Here's how the part is built. I have some questions about the finished solid (model axes, mm). Face numbers are marked on the shaded views. A direction names the side the tool comes from. Round coordinates to 2 decimals unless told otherwise and drop trailing zeros. Order: outer loops, then holes, each group sorted by start corner. A loop starts at its lowest first (then second) coordinate and runs counter-clockwise, first axis right, second up.
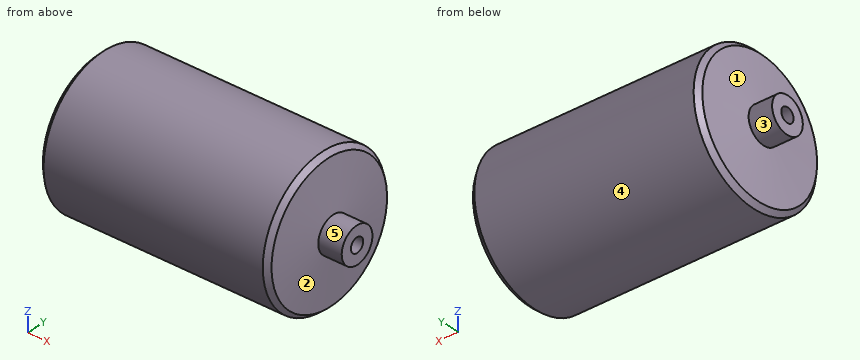
```python
from build123d import *
from OCP.BRepFilletAPI import BRepFilletAPI_MakeChamfer

# Parameters (mm, degrees)
CHAMFER1_SIZE              = 3
CHAMFER1_SIZE2             = 3.300188603
F_10_0MM_DOWEL_HOLE1_D     = 10
F_10_0MM_DOWEL_HOLE1_DEPTH = 59
F_10_0MM_DOWEL_HOLE1_TIP   = 3.004303095
F_10_0MM_DOWEL_HOLE2_D     = 10
F_10_0MM_DOWEL_HOLE2_DEPTH = 59
F_10_0MM_DOWEL_HOLE2_TIP   = 3.004303095


with BuildPart() as part:
    # Sketch1 → Revolve1 (revolve)
    with BuildSketch(Plane.XY, mode=Mode.PRIVATE) as revolve1_sk:
        Polygon((-96.096096096, 28.340840841), (103.903903904, 28.340840841), (103.903903904, 40.840840841), (87.403903904, 40.840840841), (84.123079022, 78.340840841), (-76.315271214, 78.340840841), (-79.596096096, 40.840840841), (-96.096096096, 40.840840841), align=None)
    revolve(revolve1_sk.sketch.rotate(Axis((-96.096096096, 28.340840841, 0), (1, 0, 0)), 90), axis=Axis((-96.096096096, 28.340840841, 0), (1, 0, 0)))

    # Chamfer1: one chamfer whose edges measure the first distance from different faces: ONE call of the kernel's chamfer builder (chamfer() names one face for all edges)
    chamfer1_edges_1 = [part.edges().sort_by_distance(p)[0] for p in [
        (-76.315271214, 28.340840841, -50),
    ]]
    chamfer1_side_1 = [part.faces().sort_by_distance(p)[0] for p in [
        (3.903903904, 28.340840841, -50),
    ]]
    chamfer1_edges_2 = [part.edges().sort_by_distance(p)[0] for p in [
        (84.123079022, 28.340840841, -50),
    ]]
    chamfer1_side_2 = [part.faces().sort_by_distance(p)[0] for p in [
        (85.763491463, 28.340840841, -31.25),
    ]]
    chamfer1 = BRepFilletAPI_MakeChamfer(part.part.solid().wrapped)
    for e in chamfer1_edges_1:
        chamfer1.Add(CHAMFER1_SIZE, CHAMFER1_SIZE2, e.wrapped, chamfer1_side_1[0].wrapped)  # the first distance lies on this face
    for e in chamfer1_edges_2:
        chamfer1.Add(CHAMFER1_SIZE, CHAMFER1_SIZE2, e.wrapped, chamfer1_side_2[0].wrapped)  # the first distance lies on this face
    add(Compound.cast(chamfer1.Shape()), mode=Mode.REPLACE)

    # 10.0mm Dowel Hole1
    with Locations(Plane(origin=(103.903903904, 0, 0), x_dir=(0, 0, -1), z_dir=(1, 0, 0))):
        with Locations((0, 28.340840841)):
            Hole(F_10_0MM_DOWEL_HOLE1_D / 2, depth=F_10_0MM_DOWEL_HOLE1_DEPTH)
            with Locations((0, 0, -(F_10_0MM_DOWEL_HOLE1_DEPTH + F_10_0MM_DOWEL_HOLE1_TIP / 2))):  # 118° drill point
                Cone(0, F_10_0MM_DOWEL_HOLE1_D / 2, F_10_0MM_DOWEL_HOLE1_TIP, mode=Mode.SUBTRACT)

    # 10.0mm Dowel Hole2
    with Locations(Plane.ZY.offset(96.096096096)):
        with Locations((0, 28.340840841)):
            Hole(F_10_0MM_DOWEL_HOLE2_D / 2, depth=F_10_0MM_DOWEL_HOLE2_DEPTH)
            with Locations((0, 0, -(F_10_0MM_DOWEL_HOLE2_DEPTH + F_10_0MM_DOWEL_HOLE2_TIP / 2))):  # 118° drill point
                Cone(0, F_10_0MM_DOWEL_HOLE2_D / 2, F_10_0MM_DOWEL_HOLE2_TIP, mode=Mode.SUBTRACT)


solid = part.part
```
1. If we section it at A-A, the plane x = -61.5: Write out the boundary of the cut face in (y, z).
Evaluation:
outline: circle Ø100 at (28.34, 0); hole circle Ø10 at (28.34, 0)
2. On a 3-axis mill with a long thin cutter (end or side, diameter ignored), from which of +Z, -Z, +X, -X, +Y, -Y can I reach the whole of each face in a straight line? I mean the marked faces 4 and 5. Say none if no direction works.
Evaluation:
face 4: +X, -X
face 5: +X
3. I'm going to push flat-ended pins straight in: P1, Ø8, axis at y = 28.34, z = 0, coming from the +X side; P2, Ø1, axis at x = 30, y = -9, coming from the -Z side; P3, Ø5, axis at x = 36.5, y = 62.5, coming from the +Z side; P4, Ø4, axis at x = 1, y = 29, coming from the -Z side. Where does each tip first touch, or does it pass through?
Evaluation:
P1: stops at x = 44.3
P2: stops at z = -33.8
P3: stops at z = 38.7
P4: stops at z = -50
4. I need wall thicknesses on probe 1 along Y at (x, z) = (-81, 0); probe 2 along Y at (x, z) = (81, 0); probe 3 along Z at (x, y) = (-42, 11). Which ranges of each line are inside material? Lowest first, please.
Evaluation:
probe 1: y = 15.84 to 23.34, 33.34 to 40.84
probe 2: y = -21.51 to 23.34, 33.34 to 78.19
probe 3: z = -46.9 to 46.9
5. If we mould it in two halves opening along X, with no side actions, what happens to the marked faces 1, 2 and 3? For each: released by +X, released by -X, zero draft, split by the parting line, or undercut.
Evaluation:
face 1: released by -X
face 2: released by +X
face 3: zero draft
6. If we section it at B-B, the plane x = -32: Write out the boundary of the cut face in (y, z), and give its area (3 significant figures).
Evaluation:
outline: circle Ø100 at (28.34, 0)
area: 7,850 mm2
